Geometry check sheet. Reference: drawing and pictorial views, mm from the part's lowest x, y, z. A direction names the side the tool comes from. Coordinates: 2 decimals unless noted, no trailing zeros. Loops run counter-clockwise (first coordinate to the right, second up) from the corner with the lowest first, then second, coordinate; pieces in that order, holes last. Notation, with made-up numbers: (-24.75, 6) -> (22.25, 6) arc R21 ccw to (22.25, 30) -> close; hole circle Ø10 at (15.25, 72.5). An arc over 180 degrees is marked (long way). Use one line per item in the form item = value.
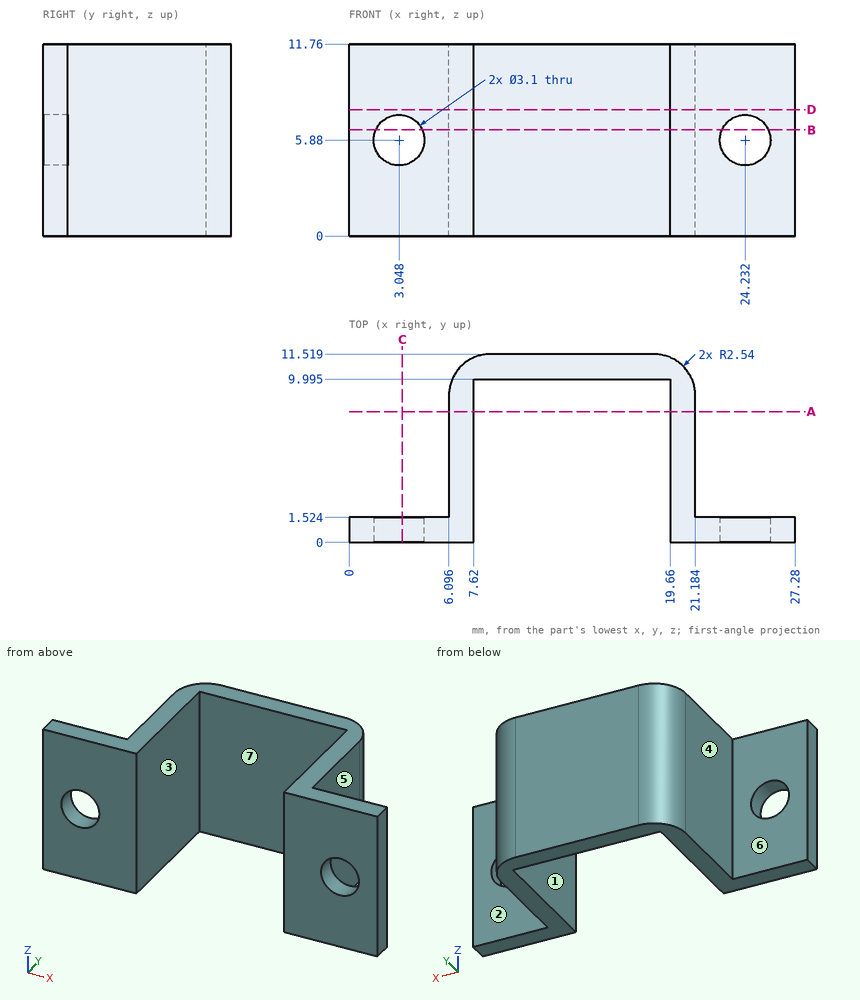
(1) Tool access check on the marked faces 5, 6 and 7. Record the directions out of +Z, -Z, +X, -X, +Y, -Y that give a thin tool (end or side, any length) a straight path to the whole face; none if there is none.
Established:
face_5 = +Z, -Z, +X, +Y
face_6 = +Z, -Z, -X, +Y
face_7 = +Z, -Z, -Y
(2) Mould release check, pull along X, two halves, no side actions. Record for the marked faces 1, 2, 3 and 4: +X half, -X half, draft (parallel to the pull), parting line (faces both ways), or undercut.
Established:
face_1 = undercut
face_2 = draft
face_3 = undercut
face_4 = -X half
(3) Section check A-A, the plane y = 8. Record the boundary of the cut face in (x, z).
Established:
outline = (6.1, 0) -> (7.62, 0) -> (7.62, 11.76) -> (6.1, 11.76) -> close; (19.66, 0) -> (21.18, 0) -> (21.18, 11.76) -> (19.66, 11.76) -> close
(4) Section check C-C, the plane x = 3.25. Record the boundary of the cut face in (y, z).
Established:
outline = (0, 0) -> (1.52, 0) -> (1.52, 4.34) -> (0, 4.34) -> close; (0, 7.42) -> (1.52, 7.42) -> (1.52, 11.76) -> (0, 11.76) -> close
(5) Scan lines: line 1 along X through (y, z) = (4.75, 3.75); line 2 along Y through (x, z) = (2.75, 9.75); line 3 along Y through (x, z) = (11.25, 2) (1 decimal). Record each from-to range of solid material in increasing order.
Established:
line_1 = 6.1 to 7.62, 19.66 to 21.18
line_2 = 0 to 1.52
line_3 = 10 to 11.5
(6) Section check D-D, the plane z = 7.75. Record the boundary of the cut face in (x, y) (1 decimal).
Established:
outline = (0, 0) -> (7.6, 0) -> (7.6, 10) -> (19.7, 10) -> (19.7, 0) -> (27.3, 0) -> (27.3, 1.5) -> (21.2, 1.5) -> (21.2, 9) arc R2.5 ccw to (18.6, 11.5) -> (8.6, 11.5) arc R2.5 ccw to (6.1, 9) -> (6.1, 1.5) -> (0, 1.5) -> close
(7) Go/stop test with flat-tipped pins: P1, Ø3, axis at x = 23.5, z = 3.5, coming from the +Y side; P2, Ø5, axis at y = 6.5, z = 3.5, coming from the -X side; P3, Ø5, axis at y = 10, z = 3.5, coming from the +X side. Record where each tip stops, or that it passes through.
Established:
P1 = 1.52
P2 = 6.1
P3 = 21.18
(8) Section check B-B, the plane z = 6.5. Record the boundary of the cut face in (x, y) (1 decimal).
Established:
outline = (0, 0) -> (1.6, 0) -> (1.6, 1.5) -> (0, 1.5) -> close; (4.5, 0) -> (7.6, 0) -> (7.6, 10) -> (19.7, 10) -> (19.7, 0) -> (22.8, 0) -> (22.8, 1.5) -> (21.2, 1.5) -> (21.2, 9) arc R2.5 ccw to (18.6, 11.5) -> (8.6, 11.5) arc R2.5 ccw to (6.1, 9) -> (6.1, 1.5) -> (4.5, 1.5) -> close; (25.7, 0) -> (27.3, 0) -> (27.3, 1.5) -> (25.7, 1.5) -> close
